Part print with two shaded views. Sizes in mm from the minimum x, y, z corner. A direction names the side the tool comes from. Coordinates: 2 decimals unless noted, no trailing zeros. Order: outer loops, then holes, each group sorted by start corner. A loop starts at its lowest first (then second) coordinate and runs counter-clockwise, first axis right, second up.
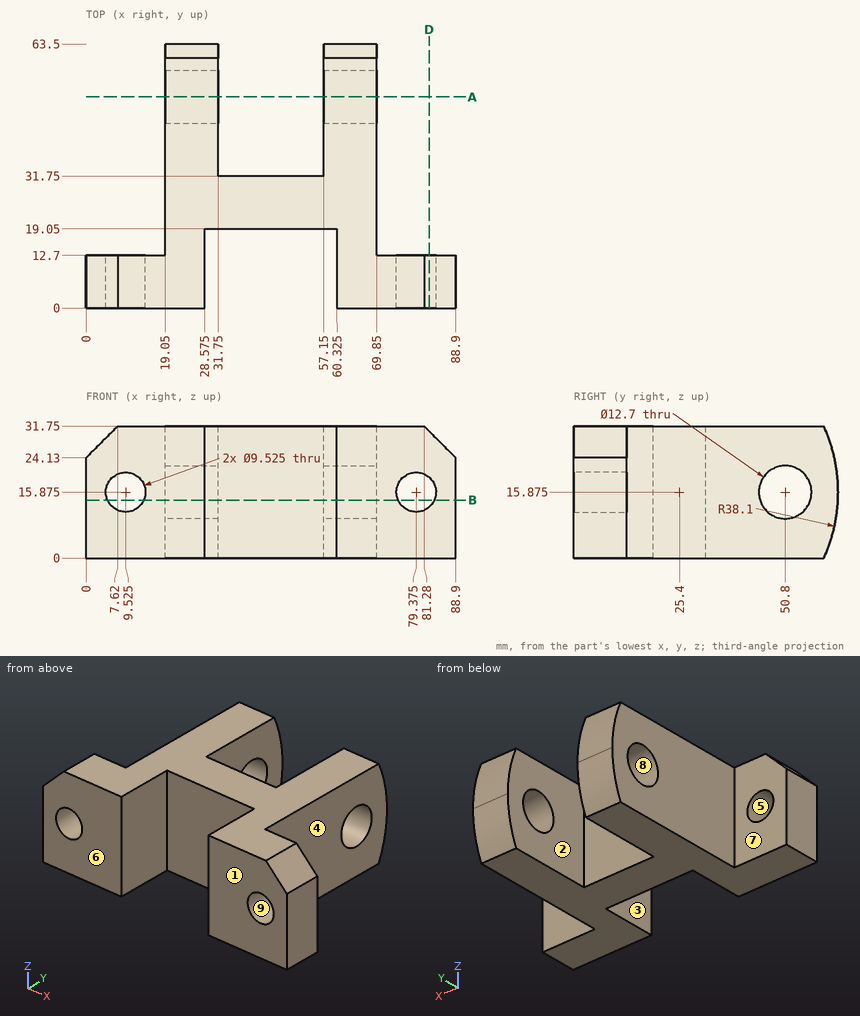
Q1. Cut at B-B on z = 14. Count the separate pieces of the cut face and the enclosed holes in it, and give its area (3 significant figures).
Results list:
separate pieces: 5
enclosed holes: 0
area: 1,770 mm2
Q2. Cut at D-D on x = 82.5. Write the cut outline in (y, z), and give its area (3 significant figures).
Results list:
outline: (0, 0) - (12.7, 0) - (12.7, 12.28) - (0, 12.28) - close; (0, 19.47) - (12.7, 19.47) - (12.7, 30.53) - (0, 30.53) - close
area: 296 mm2
Q3. Wall check: line 1 along X through (y, z) = (17, 24) (3 decimals); line 2 along X through (y, z) = (36, 5.5); line 3 along X through (y, z) = (4.5, 15) (3 decimals). Give the ranges that are in metal, low to high.
Results list:
line 1: x = 19.05 to 28.575, 60.325 to 69.85
line 2: x = 19.05 to 31.75, 57.15 to 69.85
line 3: x = 0 to 4.844, 14.206 to 28.575, 60.325 to 74.694, 84.056 to 88.9
Q4. Cut at A-A on y = 50.8. Write the cut outline in (x, z) (3 decimals).
Results list:
outline: (19.05, 0) - (31.75, 0) - (31.75, 9.525) - (19.05, 9.525) - close; (19.05, 22.225) - (31.75, 22.225) - (31.75, 31.75) - (19.05, 31.75) - close; (57.15, 0) - (69.85, 0) - (69.85, 9.525) - (57.15, 9.525) - close; (57.15, 22.225) - (69.85, 22.225) - (69.85, 31.75) - (57.15, 31.75) - close
Q5. Mould opens along Y. For the marked faces 6, 7, 8 and 9 say: pulls with the +Y half, pulls with the -Y half, needs draft (parallel to the pull), parting line crosses it, or undercut.
Results list:
face 6: pulls with the -Y half
face 7: pulls with the +Y half
face 8: undercut
face 9: needs draft
Q6. Pin check, flat tips, straight feed: pin 1 Ø1 at (y, z) = (26, 22) entering from -X; pin 2 Ø8.5 at (x, z) = (9.525, 15.875) entering from -Y; pin 3 Ø8 at (x, z) = (66, 28) entering from +Y; pin 4 Ø15 at (x, z) = (8, 13) entering from +Y. Stop position of each tip, or through.
Results list:
pin 1: stops at x = 19.05
pin 2: passes through
pin 3: stops at y = 62.62
pin 4: stops at y = 12.7
Q7. Which spindle directions (+Z, -Z, +X, -X, +Y, -Y) get a long thin tool onto all of the face, cutting with end or side? Do the marked faces 1, 2, 3, 4 and 5. Say none if no direction does.
Results list:
face 1: +Z, -Z, +X, -X, -Y
face 2: +Z, -Z, +Y
face 3: +Z, -Z, -Y
face 4: +Z, -Z, +X, +Y
face 5: +Y, -Y
